from build123d import *

# Parameters (mm, degrees)
F2_SIZE  = 0.5
F5_DEPTH = 1.5


with BuildPart() as f1:
    # F0 (on Front) → F1 (revolve)
    with BuildSketch(Plane.XZ):
        with BuildLine():
            Line((0, 12), (0, 0))
            Line((0, 0), (1.5, 0))
            Line((1.5, 0), (1.5, 10))
            Line((1.5, 10), (3, 10))
            ThreePointArc((3, 10), (1.802776, 11.454163), (0, 12))
        make_face()
    revolve(axis=Axis((0, 0, 6), (0, 0, 1)))

    # F2
    f2_edges = [f1.edges().sort_by_distance(p)[0] for p in [
        (-1.5, 0, 0),
    ]]
    chamfer(f2_edges, length=F2_SIZE)

    # F4 (on offset) → F5 (cut)
    with BuildSketch(Plane.XY.offset(12)):
        Polygon((0.57735, 1), (-0.57735, 1), (-1.154701, 0), (-0.57735, -1), (0.57735, -1), (1.154701, 0), align=None)
    extrude(amount=-F5_DEPTH, mode=Mode.SUBTRACT)


solid = f1.part
Model file for the job. Use its own axes, mm. A direction names the side the tool comes from. Round coordinates to 2 decimals unless told otherwise and drop trailing zeros. Order: outer loops, then holes, each group sorted by start corner. A loop starts at its lowest first (then second) coordinate and runs counter-clockwise, first axis right, second up.
(1) Drill centre lines: line 1 (Y direction, x = 0, z = 7.75); line 2 (Z direction, x = 0.5, y = 0.25); line 3 (X direction, y = -1, z = 8.25). Where is each one in solid material? Low to high.
(2) Band-saw the part on A-A (z = 5). List the corners of the cut face in (x, y), then the cut area to 3 significant figures.
(3) Pin check, flat tips, straight feed: pin 1 (0.9 mm diameter, centred on x = -0.5, z = 11, fed in from -Y); pin 2 (1.3 mm diameter, centred on x = 0, z = 11.5, fed in from +Y); pin 3 (1.5 mm diameter, centred on x = -1.5, z = 7, fed in from +Y). Stop position of each tip, or through.
(4) 3-axis set-ups, long thin cutter, end or side, ignore diameter. For faces 4 (the face through (0, 0, 0)), 5 (the face through (0, -1, 11)): which of +Z, -Z, +X, -X, +Y, -Y reach the whole face in a straight line?
(5) Pull direction X, two halves, no side cores. Call faces 1 (the face through (0.86, -0.51, 11.18)), 2 (the face through (-1.3, -1.3, 10)), 3 (the face through (-1.5, 0.07, 5.32)): released by +X, released by -X, zero draft, split by the parting line, or undercut.
Verdict:
1. line 1: y = -1.5 to 1.5
1. line 2: z = 0 to 10.5
1. line 3: x = -1.12 to 1.12
2. outline: circle Ø3 at (0, 0)
2. area: 7.07 mm2
3. pin 1: stops at y = -2.67
3. pin 2: stops at y = 2.48
3. pin 3: stops at y = 1.3
4. face 4: -Z, +X, -X, +Y, -Y
4. face 5: +Z
5. face 1: undercut
5. face 2: zero draft
5. face 3: split by the parting line
